Here's how the part is built. I have some questions about the finished solid (model axes, mm). A direction names the side the tool comes from. Coordinates: 2 decimals unless noted, no trailing zeros. Write each loop counter-clockwise with the first axis right and the second up, starting at its lowest first coordinate (ties: lowest second). Pieces come first, ordered by that corner, then holes.
Item 1: If we mould it in two halves opening along Z, with no side actions, what happens to faces 1 (the face through (8, 4, -5.5)), 2 (the face through (54.25, 4, -5)), 3 (the face through (28, 1.6, -16)), 4 (the face through (55.14, 0.79, -40.1))? For each: pulls with the +Z half, pulls with the -Z half, needs draft (parallel to the pull), parting line crosses it, or undercut.
Item 2: I want a section at A-A (z = -29.5). Please give me the cut outline in (x, y).
Item 3: For faces 5 (the face through (15.511, 5, -34)), 6 (the face through (4.748, 5.848, -10.913)), 7 (the face through (46, 6, -32)), 8 (the face through (2.2, 4, -37)), which set-ups out of +Z, -Z, +X, -X, +Y, -Y let a thin tool reach every point of the face, with its end or its side?
Item 4: Please list where these lines run through material, in increasing order: line 1 (X direction, y = 4.25, z = -38); line 2 (X direction, y = 1.75, z = -4); line 3 (Z direction, x = 5, y = 2.5).
Item 5: I'm going to push flat-ended pins straight in: P1, Ø4.5, axis at x = 44, z = -37.5, coming from the -Y side; P2, Ø2, axis at y = 6.5, z = -33, coming from the -X side; P3, Ø11, axis at x = 29.5, z = -36.5, coming from the +Y side; P4, Ø5, axis at y = 5, z = -20.5, coming from the +X side. Where does each tip first touch, or does it pass through?
Item 6: I want a section at B-B (x = 11). Please give me the cut outline in (y, z).
Item 7: I want a section at C-C (y = 3.5). Count the separate pieces of the cut face and the enclosed holes in it, and give its area (3 significant figures).
Item 8: I want a section at D-D (z = -7). Please give me the cut outline in (x, y).
from build123d import *

# Parameters (mm, degrees)
BOSS_EXTRUDE1_DEPTH      = 1.6
BOSS_EXTRUDE2_DEPTH      = 9.1
BOSS_EXTRUDE2_DEPTH_BACK = 0.7
BOSS_EXTRUDE3_START      = 1.6
SKETCH1_4_W              = 22.1
SKETCH1_4_H              = 13.9
SKETCH1_4_W_2            = 13.15
SKETCH1_4_H_2            = 10.2
BOSS_EXTRUDE3_DEPTH      = 6.5
BOSS_EXTRUDE4_START      = 1.6
SKETCH1_5_W              = 9.1
SKETCH1_5_H              = 7.5
SKETCH1_5_W_2            = 14
SKETCH1_5_H_2            = 6.55
BOSS_EXTRUDE4_DEPTH      = 5
SKETCH2_W                = 10.965284592
SKETCH2_H                = 1.785046329
CUT_EXTRUDE1_DEPTH       = 9
SKETCH3_W                = 5.100132369
SKETCH3_H                = 1.23427986
SKETCH3_W_2              = 14.280370632
SKETCH3_H_2              = 7.586446898
CUT_EXTRUDE2_DEPTH       = 12
FILLET1_R                = 2.5


with BuildPart() as part:
    # Sketch1 → Boss-Extrude1 (new body)
    with BuildSketch(Plane(origin=(0, 0, 0), x_dir=(1, 0, 0), z_dir=(0, 1, 0))):
        with BuildLine():
            ThreePointArc((0, 3), (0.878679656, 0.878679656), (3, 0))
            Line((3, 0), (53, 0))
            ThreePointArc((53, 0), (55.121320344, 0.878679656), (56, 3))
            Line((56, 3), (56, 38))
            ThreePointArc((56, 38), (55.121320344, 40.121320344), (53, 41))
            Line((53, 41), (3, 41))
            ThreePointArc((3, 41), (0.878679656, 40.121320344), (0, 38))
            Line((0, 38), (0, 3))
        make_face()
    extrude(amount=BOSS_EXTRUDE1_DEPTH)

    # Sketch1<3> → Boss-Extrude2 (add, two sides: drawn at the far end of the back side and taken through both)
    with BuildSketch(Plane(origin=(0, 0, 0), x_dir=(1, 0, 0), z_dir=(0, 1, 0)).offset(-BOSS_EXTRUDE2_DEPTH_BACK)):
        with BuildLine():
            Line((37.95, 12.5), (37.95, 0))
            Line((37.95, 0), (53, 0))
            ThreePointArc((53, 0), (53.639713183, 0.068998969), (54.25, 0.272821971))
            Line((54.25, 0.272821971), (54.25, 12.5))
            Line((54.25, 12.5), (37.95, 12.5))
        make_face()
        with BuildLine():
            Line((53, 0), (37.95, 0))
            Line((37.95, 0), (37.95, -2))
            Line((37.95, -2), (54.25, -2))
            Line((54.25, -2), (54.25, 0.272821971))
            ThreePointArc((54.25, 0.272821971), (53.639713183, 0.068998969), (53, 0))
        make_face()
    extrude(amount=BOSS_EXTRUDE2_DEPTH + BOSS_EXTRUDE2_DEPTH_BACK)

    # Sketch1<4> → Boss-Extrude3 (add)
    with BuildSketch(Plane(origin=(0, 0, 0), x_dir=(1, 0, 0), z_dir=(0, 1, 0)).offset(BOSS_EXTRUDE3_START)):
        with Locations((26.561479759, 34.05)):
            Rectangle(SKETCH1_4_W, SKETCH1_4_H)
        with Locations((46.025, 35.9)):
            Rectangle(SKETCH1_4_W_2, SKETCH1_4_H_2)
    extrude(amount=BOSS_EXTRUDE3_DEPTH)

    # Sketch1<5> → Boss-Extrude4 (add)
    with BuildSketch(Plane(origin=(0, 0, 0), x_dir=(1, 0, 0), z_dir=(0, 1, 0)).offset(BOSS_EXTRUDE4_START)):
        with Locations((7.8, 1.75)):
            Rectangle(SKETCH1_5_W, SKETCH1_5_H)
        with Locations((4.65, 13.475)):
            Rectangle(SKETCH1_5_W_2, SKETCH1_5_H_2)
        with BuildLine():
            ThreePointArc((3, 41), (2.596328956, 40.972717559), (2.2, 40.891366459))
            Line((2.2, 40.891366459), (2.2, 33.2))
            Line((2.2, 33.2), (13.5, 33.2))
            Line((13.5, 33.2), (13.5, 41))
            Line((13.5, 41), (3, 41))
        make_face()
    extrude(amount=BOSS_EXTRUDE4_DEPTH)

    # Sketch2 → Cut-Extrude1 (cut)
    with BuildSketch(Plane(origin=(0, 0, -41), x_dir=(-1, 0, 0), z_dir=(0, 0, -1))):
        with Locations((-45.98237221, 5.889418847)):
            Rectangle(SKETCH2_W, SKETCH2_H)
    extrude(amount=-CUT_EXTRUDE1_DEPTH, mode=Mode.SUBTRACT)

    # Sketch3 → Cut-Extrude2 (cut)
    with BuildSketch(Plane.XY.offset(2)):
        with Locations((46.492385447, -0.08286007)):
            Rectangle(SKETCH3_W, SKETCH3_H)
        with Locations((46.237378828, 4.327503309)):
            Rectangle(SKETCH3_W_2, SKETCH3_H_2)
    extrude(amount=-CUT_EXTRUDE2_DEPTH, mode=Mode.SUBTRACT)

    # Fillet1
    fillet1_edges = [part.edges().sort_by_distance(p)[0] for p in [
        (-1.175, 1.6, -16.75),
        (-1.175, 1.6, -10.2),
        (4.65, 6.6, -16.75),
        (4.65, 6.6, -10.2),
    ]]
    fillet(fillet1_edges, radius=FILLET1_R - 0.0001)  # a hair under: the kernel refuses the full size


solid = part.part
Answer:
1. face 1: undercut
1. face 2: needs draft
1. face 3: undercut
1. face 4: pulls with the -Z half
2. outline: (0, 0) - (56, 0) - (56, 1.6) - (37.61, 1.6) - (37.61, 8.1) - (15.51, 8.1) - (15.51, 1.6) - (0, 1.6) - close
3. face 5: +Z, -Z, +Y
3. face 6: -X, +Y
3. face 7: -Z
3. face 8: -Z, -X, +Y
4. line 1: x = 2.2 to 13.5, 15.51 to 37.61, 39.45 to 52.6
4. line 2: x = 3.25 to 12.35, 37.95 to 39.1, 53.38 to 54.25
4. line 3: z = -41 to -33.2, -16.75 to -10.2, -5.5 to 2
5. P1: stops at y = 0
5. P2: stops at x = 2.2
5. P3: stops at y = 8.1
5. P4: passes through
6. outline: (0, -41) - (6.6, -41) - (6.6, -33.2) - (1.6, -33.2) - (1.6, -16.75) - (4.1, -16.75) arc R2.5 ccw to (6.6, -14.25) - (6.6, -12.7) arc R2.5 ccw to (4.1, -10.2) - (1.6, -10.2) - (1.6, -5.5) - (6.6, -5.5) - (6.6, 2) - (1.6, 2) - (1.6, 0) - (0, 0) - close
7. separate pieces: 6
7. enclosed holes: 0
7. area: 754 mm2
8. outline: (0, 0) - (37.95, 0) - (37.95, -0.7) - (43.94, -0.7) - (43.94, 0.53) - (39.1, 0.53) - (39.1, 8.12) - (53.38, 8.12) - (53.38, 0.53) - (49.04, 0.53) - (49.04, -0.7) - (54.25, -0.7) - (54.25, 0) - (56, 0) - (56, 1.6) - (54.25, 1.6) - (54.25, 9.1) - (37.95, 9.1) - (37.95, 1.6) - (0, 1.6) - close
